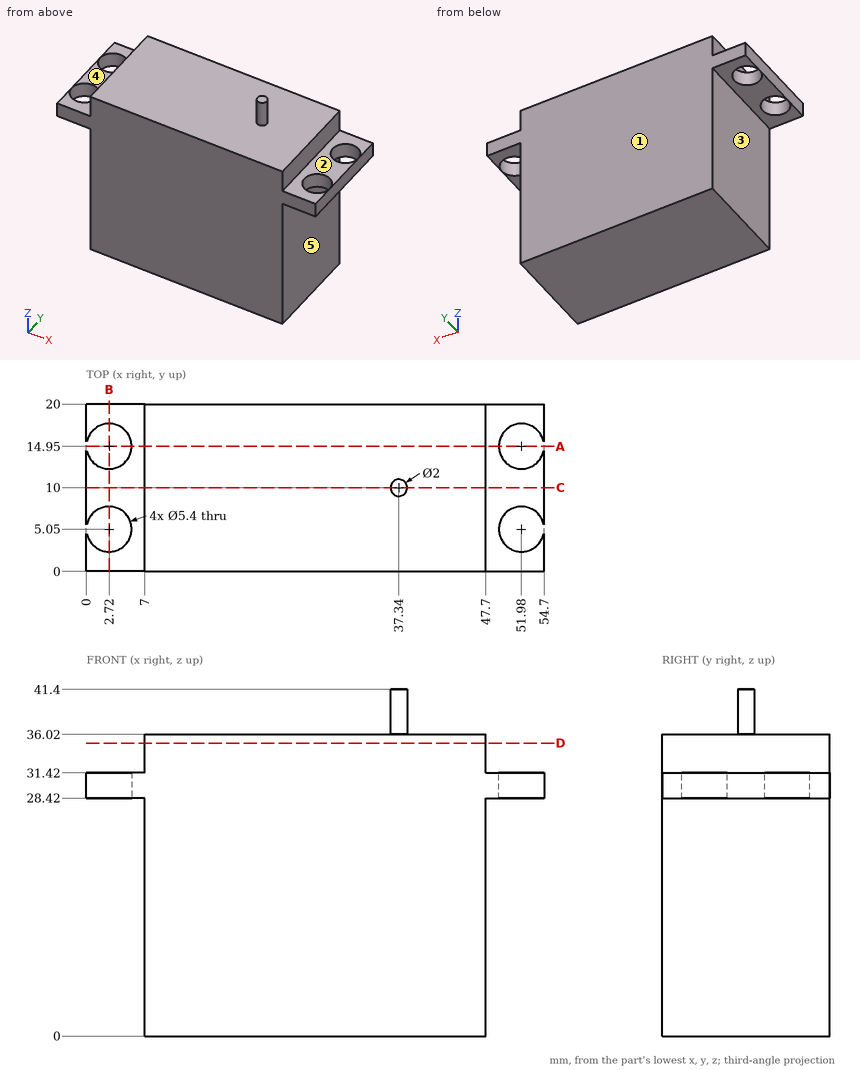
Geometry check sheet. Reference: drawing and pictorial views, mm from the part's lowest x, y, z. A direction names the side the tool comes from. Round coordinates to 2 decimals unless told otherwise and drop trailing zeros. Loops run counter-clockwise (first coordinate to the right, second up) from the corner with the lowest first, then second, coordinate; pieces in that order, holes last.
1. Gauge pin test, flat ends, axial feed: pin 1 Ø6 at (x, z) = (36, 20) entering from -Y; pin 2 Ø3 at (y, z) = (2.5, 17) entering from -X; pin 3 Ø4 at (y, z) = (4.5, 36.5) entering from +X; pin 4 Ø8.5 at (x, y) = (51.98, 14.95) entering from +Z. Record the tip position at first contact, or that the pin passes through.
2. Sectioned sample at B-B on x = 2.72. Record the boundary of the cut face in (y, z), and give its area (3 significant figures).
3. Sectioned sample at C-C on y = 10. Record the boundary of the cut face in (x, z).
4. Scan lines: probe 1 along Y at (x, z) = (2.72, 30.5); probe 2 along Y at (x, z) = (51, 29); probe 3 along Z at (x, y) = (17, 6.5). Record each from-to range of solid material in increasing order.
5. Sectioned sample at A-A on y = 14.95. Give the number of separate pieces and of enclosed holes in the cut face, and give its area (3 significant figures).
6. Sectioned sample at D-D on z = 35. Record the boundary of the cut face in (x, y).
7. Set-up check for the marked faces 1, 2, 3, 4 and 5: record each of +Z, -Z, +X, -X, +Y, -Y from which the full face is reachable in a straight line by a thin tool's end or side.
Recorded:
1. pin 1: stops at y = 0
1. pin 2: stops at x = 7
1. pin 3: stops at x = 47.7
1. pin 4: stops at z = 31.42
2. outline: (0, 28.42) - (2.35, 28.42) - (2.35, 31.42) - (0, 31.42) - close; (7.75, 28.42) - (12.25, 28.42) - (12.25, 31.42) - (7.75, 31.42) - close; (17.65, 28.42) - (20, 28.42) - (20, 31.42) - (17.65, 31.42) - close
2. area: 27.6 mm2
3. outline: (0, 28.42) - (7, 28.42) - (7, 0) - (47.7, 0) - (47.7, 28.42) - (54.7, 28.42) - (54.7, 31.42) - (47.7, 31.42) - (47.7, 36.02) - (38.34, 36.02) - (38.34, 41.4) - (36.34, 41.4) - (36.34, 36.02) - (7, 36.02) - (7, 31.42) - (0, 31.42) - close
4. probe 1: y = 0 to 2.35, 7.75 to 12.25, 17.65 to 20
4. probe 2: y = 0 to 2.53, 7.57 to 12.43, 17.47 to 20
4. probe 3: z = 0 to 36.02
5. separate pieces: 3
5. enclosed holes: 0
5. area: 1,480 mm2
6. outline: (7, 0) - (47.7, 0) - (47.7, 20) - (7, 20) - close
7. face 1: +Z, -Z, +X, -X, +Y
7. face 2: +Z, +X, +Y, -Y
7. face 3: -Z, -X, +Y, -Y
7. face 4: +Z, -X, +Y, -Y
7. face 5: -Z, +X, +Y, -Y
